```python
from build123d import *

# Parameters (mm, degrees)
SKETCH_1_R                   = 16.5
EXTRUDE_1_DEPTH              = 20
SKETCH_2_R                   = 13.75
EXTRUDE_2_DEPTH              = 30
SKETCH_3_R                   = 14.5
EXTRUDE_3_DEPTH              = 11
SKETCH_4_W                   = 9
SKETCH_4_H                   = 5
CUT_EXTRUDE_1_DEPTH          = 0.5
WRAP_1_OUTLINE_W             = 2.1
WRAP_1_OUTLINE_H             = 0.3
WRAP_1_OUTLINE_W_2           = 0.5
WRAP_1_DEPTH                 = 0.2
SKETCH_6_R                   = 1.25
CUT_EXTRUDE_2_DEPTH          = 6
CUT_EXTRUDE_3_DEPTH          = 0.5
SKETCH_8_R                   = 5
EXTRUDE_4_DEPTH              = 2.5
SKETCH_9_R                   = 3
CUT_EXTRUDE_4_DEPTH          = 2
SKETCH_10_R                  = 2.5
EXTRUDE_5_DEPTH              = 11.5
CUT_EXTRUDE_START            = -7
CUT_EXTRUDE_5_DEPTH          = 7
HOLE_WIZARD_M3_1_D           = 2.5
HOLE_WIZARD_M3_1_DEPTH       = 10
HOLE_WIZARD_M3_1_CSINK_D     = 3.4
HOLE_WIZARD_M3_1_CSINK_ANGLE = 45
HOLE_WIZARD_M3_1_TIP         = 0.751075774


# Read off the part's stored shape, not the designer's step: 包覆1
with BuildPart() as part:
    # 草图1 → 凸台-拉伸1 (new body)
    with BuildSketch(Plane(origin=(0, 0, 0), x_dir=(0, 0, -1), z_dir=(1, 0, 0))):
        Circle(SKETCH_1_R)
    extrude(amount=EXTRUDE_1_DEPTH)

    # 草图2 → 凸台-拉伸2 (add)
    with BuildSketch(Plane(origin=(20, 0, 0), x_dir=(0, 0, -1), z_dir=(1, 0, 0))):
        Circle(SKETCH_2_R)
    extrude(amount=EXTRUDE_2_DEPTH)

    # 草图3 → 凸台-拉伸3 (add)
    with BuildSketch(Plane(origin=(50, 0, 0), x_dir=(0, 0, -1), z_dir=(1, 0, 0))):
        Circle(SKETCH_3_R)
    extrude(amount=EXTRUDE_3_DEPTH)

    # 草图4 → 切除-拉伸1 (cut)
    with BuildSketch(Plane(origin=(61, 0, 0), x_dir=(0, 0, -1), z_dir=(1, 0, 0))):
        with Locations((0, 6)):
            Rectangle(SKETCH_4_W, SKETCH_4_H)
    extrude(amount=-CUT_EXTRUDE_1_DEPTH, mode=Mode.SUBTRACT)

    # 包覆1 outline → 包覆1 (add)
    # profile 1 of 6: a face of its own
    with BuildSketch(Plane(origin=(60.5, 0, 0), x_dir=(0, 0, -1), z_dir=(1, 0, 0))):
        Polygon((-2.789418513, 5.369902097), (-2.320955301, 5.52689379), (-2.003204114, 5.844644976), (-1.916544699, 6.105251187), (-1.916544699, 5.562687896), (-2.069140625, 4.810383703), (-2.217340783, 4.515867286), (-2.354865506, 4.371434929), (-2.798210047, 4.225746638), (-3.092726464, 4.225746638), (-3.52727947, 4.371434929), (-3.675479628, 4.664067445), (-3.737020372, 4.628273339), (-3.580028679, 4.312406052), (-3.103401899, 4.159810127), (-2.789418513, 4.159810127), (-2.320955301, 4.312406052), (-2.15580004, 4.473793513), (-1.998808347, 4.785265032), (-1.848724288, 5.55201246), (-1.848724288, 6.321899723), (-2.003204114, 6.942330894), (-2.320955301, 7.25819818), (-2.789418513, 7.415189873), (-2.950805973, 7.415189873), (-3.419269185, 7.25819818), (-3.737020372, 6.942330894), (-3.891500198, 6.473867682), (-3.891500198, 6.313108188), (-3.737020372, 5.844644976), (-3.419269185, 5.52689379), (-2.950805973, 5.369902097), align=None)
        Polygon((-2.798210047, 7.35553303), (-2.354865506, 7.209844739), (-2.064744858, 6.917212223), (-1.916544699, 6.328179391), (-2.064744858, 5.889230617), (-2.354865506, 5.599109968), (-2.798210047, 5.450281843), (-2.942014438, 5.450281843), (-3.385358979, 5.599109968), (-3.675479628, 5.889230617), (-3.823679786, 6.331947191), (-3.823679786, 6.476379549), (-3.675479628, 6.917212223), (-3.385358979, 7.209844739), (-2.942014438, 7.35553303), align=None, mode=Mode.SUBTRACT)
    # profile 2 of 6: a face of its own
    with BuildSketch(Plane(origin=(60.5, 0, 0), x_dir=(0, 0, -1), z_dir=(1, 0, 0))):
        Polygon((-1.248388054, 7.389443236), (-0.038296084, 4.2), (0.033920095, 4.2), (1.241500198, 7.375), (1.182471321, 7.400118671), (-0.002501978, 4.295450949), (-1.189359177, 7.415189873), align=None)
    # profile 3 of 6: a face of its own
    with BuildSketch(Plane(origin=(60.5, 0, 0), x_dir=(0, 0, -1), z_dir=(1, 0, 0))):
        with Locations((2.95, 6.883089037)):
            Rectangle(WRAP_1_OUTLINE_W, WRAP_1_OUTLINE_H)
    # profile 4 of 6: a face of its own
    with BuildSketch(Plane(origin=(60.5, 0, 0), x_dir=(0, 0, -1), z_dir=(1, 0, 0))):
        with Locations((3.75, 5.236905413)):
            Rectangle(WRAP_1_OUTLINE_W_2, WRAP_1_OUTLINE_H)
    # profile 5 of 6: a face of its own
    with BuildSketch(Plane(origin=(60.5, 0, 0), x_dir=(0, 0, -1), z_dir=(1, 0, 0))):
        with Locations((2.15, 5.236905413)):
            Rectangle(WRAP_1_OUTLINE_W_2, WRAP_1_OUTLINE_H)
    # profile 6 of 6: a face of its own
    with BuildSketch(Plane(origin=(60.5, 0, 0), x_dir=(0, 0, -1), z_dir=(1, 0, 0))):
        with Locations((2.95, 5.236905413)):
            Rectangle(WRAP_1_OUTLINE_W_2, WRAP_1_OUTLINE_H)
    extrude(amount=WRAP_1_DEPTH)

    # 草图6 → 切除-拉伸2 (cut)
    with BuildSketch(Plane(origin=(61, 0, 0), x_dir=(0, 0, -1), z_dir=(1, 0, 0))):
        with Locations((-7, -3)):
            Circle(SKETCH_6_R)
        with Locations(Location((7, -3, 0), (0, 0, 180))):
            Circle(SKETCH_6_R)
    extrude(amount=-CUT_EXTRUDE_2_DEPTH, mode=Mode.SUBTRACT)

    # 草图7 → 切除-拉伸3 (cut)
    with BuildSketch(Plane.ZY):
        with BuildLine():
            ThreePointArc((6.32455532, -9), (0, 11), (-6.32455532, -9))
            ThreePointArc((-6.32455532, -9), (0, 1), (6.32455532, -9))
        make_face()
    extrude(amount=-CUT_EXTRUDE_3_DEPTH, mode=Mode.SUBTRACT)

    # 草图8 → 凸台-拉伸4 (add)
    with BuildSketch(Plane.ZY):
        with Locations(Location((0, -6, 0), (0, 0, 180))):
            Circle(SKETCH_8_R)
    extrude(amount=EXTRUDE_4_DEPTH)

    # 草图9 → 切除-拉伸4 (cut)
    with BuildSketch(Plane.ZY.offset(2.5)):
        with Locations((0, -6)):
            Circle(SKETCH_9_R)
    extrude(amount=-CUT_EXTRUDE_4_DEPTH, mode=Mode.SUBTRACT)

    # 草图10 → 凸台-拉伸5 (add)
    with BuildSketch(Plane.ZY.offset(0.5)):
        with Locations((0, -6)):
            Circle(SKETCH_10_R)
    extrude(amount=EXTRUDE_5_DEPTH)

    # 草图11 → 切除-拉伸5 (cut)
    with BuildSketch(Plane.ZY.offset(12).offset(CUT_EXTRUDE_START)):
        with BuildLine():
            Line((0, -4.5), (-2, -4.5))
            ThreePointArc((-2, -4.5), (0, -3.5), (2, -4.5))
            Line((2, -4.5), (0, -4.5))
        make_face()
    extrude(amount=CUT_EXTRUDE_5_DEPTH, mode=Mode.SUBTRACT)

    # M3 螺纹孔1
    with Locations(Plane(origin=(0, 13.4, 0), x_dir=(0, 0, -1), z_dir=(-1, 0, 0))):
        with Locations((0, 0)):
            CounterSinkHole(HOLE_WIZARD_M3_1_D / 2, HOLE_WIZARD_M3_1_CSINK_D / 2, depth=HOLE_WIZARD_M3_1_DEPTH, counter_sink_angle=HOLE_WIZARD_M3_1_CSINK_ANGLE)
            with Locations((0, 0, -(HOLE_WIZARD_M3_1_DEPTH + HOLE_WIZARD_M3_1_TIP / 2))):  # 118° drill point
                Cone(0, HOLE_WIZARD_M3_1_D / 2, HOLE_WIZARD_M3_1_TIP, mode=Mode.SUBTRACT)


solid = part.part
```
Check sheet for the modelled part. Datum: model origin and axes. Units: mm. A direction names the side the tool comes from. Give positions to 0.01 mm unless a question says otherwise; leave off trailing zeros. Loops run counter-clockwise (first coordinate to the right, second up) from the corner with the lowest first, then second, coordinate; pieces in that order, holes last. Notation, with made-up numbers: M 60.25,-35.5 L 115.25,-35.5 A20 cw 115.25,-29.5 Z; hole C -23,80 d1. An arc over 180 degrees is marked long. Answer as CSV lines item,"result".
Item 1: Draft check along X on faces 6 (the face through (-1.23, -1.12, 1.08)), 7 (the face through (20, 14, 4)), 8 (the face through (-2.5, -6.1, -3.3)). Enter one of: pulls with the +X half, pulls with the -X half, needs draft (parallel to the pull), parting line crosses it, or undercut.
Reply:
face 6,"needs draft"
face 7,"undercut"
face 8,"pulls with the -X half"
Item 2: Sectioned sample at B-B, the plane z = -10. Enter the section's corners in (x, y).
Reply:
outline,"M 0,-13.12 L 20,-13.12 L 20,-9.44 L 50,-9.44 L 50,-10.5 L 61,-10.5 L 61,10.5 L 50,10.5 L 50,9.44 L 20,9.44 L 20,13.12 L 0,13.12 L 0,4.58 L 0.5,4.58 L 0.5,-4.58 L 0,-4.58 Z"
Item 3: Set-up check for faces 1 (the face through (50, -9, 11)), 2 (the face through (9.86, -6.32, -15.24)), 3 (the face through (-12, -6, 0)), 4 (the face through (58.042, -3.845, -7.921)), 5 (the face through (5.61, 14.62, -0.27)): record each of +Z, -Z, +X, -X, +Y, -Y from which the full face is reachable in a straight line by a thin tool's end or side.
Reply:
face 1,"none"
face 2,"+X, -X"
face 3,"+Z, -Z, -X, +Y, -Y"
face 4,"+X"
face 5,"-X"
Item 4: Sectioned sample at D-D, the plane x = 21. Enter the section's corners in (y, z).
Reply:
outline,"C 0,0 d27.5"
Item 5: Depth check by flat-ended pin: pin 1 Ø6 at (x, z) = (9.5, -11.5) entering from -Y; pin 2 Ø1.5 at (x, y) = (38, 8) entering from -Z; pin 3 Ø5 at (x, y) = (8.5, 3.5) entering from +Z. Enter the tip coordinate at first touch or a pass-through.
Reply:
pin 1,"y = -14.14"
pin 2,"z = -11.68"
pin 3,"z = 16.47"
Item 6: Scan lines: L1, parallel to Y at x = 5.75, z = 0; L2, parallel to X at y = -5, z = -10.5; L3, parallel to Y at x = 57, z = 7. Record each from-to range of solid material in increasing order.
Reply:
L1,"-16.5 to 12.15, 14.65 to 16.5"
L2,"0 to 61"
L3,"-12.7 to -4.25, -1.75 to 12.7"
Item 7: Sectioned sample at C-C, the plane x = 7.5. Enter the section's corners in (y, z).
Reply:
outline,"C 0,0 d33; hole C 13.4,0 d2.5"
